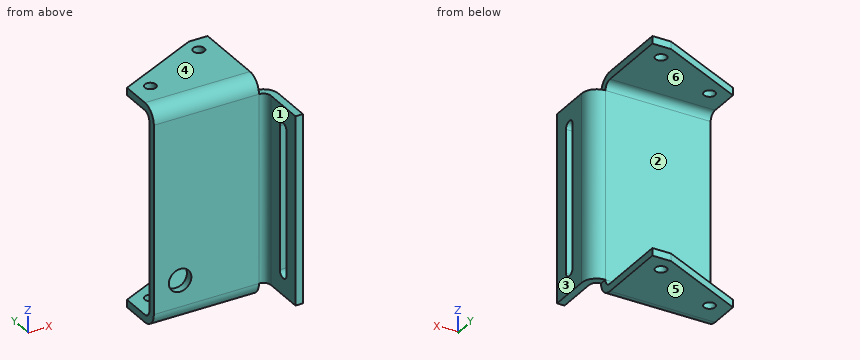
Autodesk Inventor part; units mm, degrees
ref_plane "YZ Plane" through (0, 0, 0) normal (1, 0, 0) x (0, 1, 0)
ref_plane "XZ Plane" through (0, 0, 0) normal (0, 1, 0) x (-1, 0, 0)
ref_plane "XY Plane" through (0, 0, 0) normal (0, 0, 1) x (1, 0, 0)
sketch "スケッチ1" plane through (0, 0, 0) normal (0, 1, 0) x (-1, 0, 0)
  line L0 (-14, -27) -> (14, -27)
  line L1 (14, 27) -> (-14, 27)
  line L2 (-14, 27) -> (-14, -27)
  line L3 (-14, -27) -> (14, 27) construction
  line L4 (14, -27) -> (-14, 27) construction
  line L5 (14, -27) -> (14, 27)
  point P0 (0, 0)
  dimension "d0" = 28
  dimension "d1" = 54
extrude "プレート1" add sketch "スケッチ1" along normal blind 2
sketch "スケッチ2" plane through (-14, 0, 27) normal (0, 0, 1) x (1, 0, 0)
  line L0 (0, 2) -> (28, 2)
  line L1 (0, 2) -> (0, 12)
  line L2 (0, 12) -> (23, 23)
  line L3 (23, 23) -> (28, 23)
  line L4 (28, 23) -> (28, 2)
  line L5 (0, 0) -> (0, 2)
  line L6 (28, 2) -> (0, 2)
  point P0 (14, 0)
  dimension "d3" = 10
  dimension "d4" = 5
  dimension "d5" = 21
sheet face with bend "面2" sketch "スケッチ2" thickness 2 toward (0, 0, 1) bend radius 2
bend "曲げ1"
sketch "スケッチ3" plane through (14, 0, -27) normal (0, 0, -1) x (-1, 0, 0)
  line L0 (0, 0) -> (0, 2)
  line L1 (0, 2) -> (0, 23)
  line L2 (0, 23) -> (5, 23)
  line L3 (0, 23) -> (5, 23)
  line L4 (28, 12) -> (28, 4)
  line L5 (5, 23) -> (28, 12)
  line L6 (28, 0) -> (28, 2)
  line L7 (28, 12) -> (28, 2)
  line L8 (28, 2) -> (0, 2)
  point P0 (14, 0)
sheet face with bend "面3" sketch "スケッチ3" thickness 2 toward (0, 0, -1) bend radius 2
bend "曲げ2"
sketch "スケッチ4" plane through (14, 0, -29) normal (0, 0, -1) x (-1, 0, 0)
  line L0 (5, 23) -> (28, 12)
  line L1 (0, 23) -> (5, 23)
  line L2 (28, 4) -> (28, 12)
  point P0 (14, 0)
  point P1 (4.9573, 18.5865)
  point P2 (23, 9.9574)
  dimension "d16" = 4
  dimension "d17" = 4
  dimension "d18" = 20
  dimension "d44" = 5
hole "穴1" at (9.0427, 18.5865, -29) at (-9, 9.9574, -29) direction (0, 0, 1) diameter 3 end through all
sketch "スケッチ6" plane through (16, -2, -25) normal (1, 0, 0) x (0, -1, 0)
  line L0 (0, 50) -> (0, 0)
  line L1 (0, 0) -> (11, 0)
  line L2 (11, 0) -> (11, 50)
  line L3 (11, 50) -> (0, 50)
edge flange "フランジ1" height 15 angle 90 thickness 2 bend radius 2 thickness toward (1, 0, 0) relief straight relief width 2 relief depth 1 edges at (14, 2, 0) wall of the first edge with corners at (16, -2, 25) (16, -2, -25) (16, -13, -25) (16, -13, 25)
bend "曲げ3"
corner "コーナー1"
sketch "スケッチ8" plane through (16, -13, -25) normal (-1, 0, 0) x (0, 0, 1)
  line L0 (44, 4) -> (6, 4)
  arc A0 (6, 7) -> (6, 4) centre (6, 5.5) ccw
  line L1 (6, 7) -> (44, 7)
  arc A1 (44, 4) -> (44, 7) centre (44, 5.5) ccw
  line L2 (50, 11) -> (50, 0)
  line L3 (0, 0) -> (0, 11)
  line L4 (50, 0) -> (0, 0)
  point P0 (25, 13)
  point P1 (50, 5.5)
  dimension "d66" = 6
  dimension "d67" = 6
  dimension "d69" = 1.5
extrude "押し出し2" cut sketch "スケッチ8" against normal blind 10
sketch "スケッチ9" plane through (0, 2, 0) normal (0, 1, 0) x (1, 0, 0)
  line L0 (14, 25) -> (-14, 25)
  line L1 (-14, -25) -> (-14, 25)
  point P0 (0, 0)
  point P1 (-7, 18)
  dimension "d72" = 7
  dimension "d73" = 7
hole "穴3" at (-7, 2, -18) direction (0, -1, 0) diameter 6 end through all
equation "\"d25\" = Thickness"
equation "\"d79\" = Thickness"
equation "\"d2\" = Thickness"
equation "\"d6\" = BendRadius"
equation "\"d7\" = BendReliefWidth"
equation "\"d9\" = MinimumRemnant"
equation "\"d8\" = BendReliefDepth"
equation "\"d10\" = TransitionRadius"
equation "\"d11\" = BendRadius"
equation "\"d12\" = BendReliefWidth"
equation "\"d14\" = MinimumRemnant"
equation "\"d13\" = BendReliefDepth"
equation "\"d15\" = TransitionRadius"
equation "\"d45\" = BendReliefWidth"
equation "\"d46\" = BendReliefDepth"
equation "\"d47\" = MinimumRemnant"
equation "\"d48\" = TransitionRadius"
equation "\"d51\" = BendRadius"
equation "\"d52\" = CornerReliefSize"
equation "\"d53\" = GapSize"
equation "\"d54\" = JacobiRadiusSize"
equation "\"BendRadius\" = Thickness"
equation "\"BendReliefWidth\" = Thickness"
equation "\"BendReliefDepth\" = 0.5 * Thickness"
equation "\"CornerReliefSize\" = 4 * Thickness"
equation "\"MinimumRemnant\" = 2 * Thickness"
equation "\"TransitionRadius\" = BendRadius"
equation "\"JacobiRadiusSize\" = Thickness"
equation "\"GapSize\" = Thickness"
properties part number "trackball_l" material "アルミニウム 6061"
The model under review builds one solid part; all positions refer to its coordinate system, in mm. Face numbers are marked on the shaded views. A direction names the side the tool comes from. Round coordinates to 2 decimals unless told otherwise and drop trailing zeros. Write each loop counter-clockwise with the first axis right and the second up, starting at its lowest first coordinate (ties: lowest second). Pieces come first, ordered by that corner, then holes. Notation, with made-up numbers: (35, 1.25) - (92, 1.25) arc R24 cw to (92, 25.25) - close; hole circle Ø3 at (55.25, 29). An arc over 180 degrees is marked (long way). One line per item, written item: value. Start each with the question number.
1. The part is to be moulded in two halves that separate along Z. For the marked faces 4, 5 and 6, say which applies: released by +Z, released by -Z, zero draft, split by the parting line, or undercut.
2. Consider section D-D on y = 16. Write out the cut boundary in (x, z).
3. Consider section C-C on x = 0. Write out the cut boundary in (y, z), and give its area (3 significant figures).
4. Consider section B-B on y = -7.5. Write out the cut boundary in (x, z).
5. Machinability: for the marked faces 1, 2 and 3, which of the approach directions +Z, -Z, +X, -X, +Y, -Y give a long, thin tool a straight path to every point of the face, cutting with its end or side? Answer none if there is none.
6. Clearance check with flat-ended pins moving along their axes: P1, Ø9.5, axis at x = -7, z = -18, coming from the -Y side; P2, Ø3.5, axis at x = -9, y = 9.96, coming from the +Z side; P3, Ø3, axis at y = 10, z = 28, coming from the +X side; P4, Ø1, axis at x = -4.5, z = 21, coming from the +Y side. State where each tip first meets the part, or that it passes through.
7. To check wall thickness, follow L1, parallel to Z at x = -5, y = 9; L2, parallel to Y at x = -6, z = 21.5; L3, parallel to X at y = -2.5, z = -6.5. State the ranges of each line that lie inside material, in increasing order. Write a range as from..to.
8. Consider section A-A on z = -18. Write out the cut boundary in (x, y).
Checks:
1. face 4: released by +Z
1. face 5: released by -Z
1. face 6: undercut
2. outline: (-5.64, -29) - (14, -29) - (14, -27) - (-5.64, -27) - close; (-5.64, 27) - (14, 27) - (14, 29) - (-5.64, 29) - close
3. outline: (0, -25) arc R4 ccw to (4, -29) - (18.7, -29) - (18.7, -27) - (4, -27) arc R2 cw to (2, -25) - (2, 25) arc R2 cw to (4, 27) - (18.7, 27) - (18.7, 29) - (4, 29) arc R4 ccw to (0, 25) - close
3. area: 178 mm^2
4. outline: (16, -25) - (18, -25) - (18, -20.5) - (16, -20.5) - close; (16, 20.5) - (18, 20.5) - (18, 25) - (16, 25) - close
5. face 1: +Z, -Z, -X, -Y
5. face 2: +X, -X, +Y
5. face 3: +Z, -Z, +X, +Y, -Y
6. P1: stops at y = 0
6. P2: stops at z = 29
6. P3: stops at x = 14
6. P4: stops at y = 2
7. L1: z = -29..-27, 27..29
7. L2: y = 0..2
7. L3: x = 16..18
8. outline: (-14, 0) - (-10, 0) - (-10, 2) - (-14, 2) - close; (-4, 0) - (14, 0) arc R2 cw to (16, -2) - (16, -6) - (18, -6) - (18, -2) arc R4 ccw to (14, 2) - (-4, 2) - close; (16, -13) - (18, -13) - (18, -9) - (16, -9) - close
